The drawing under review shows one solid part. Ordinate dimensions are in mm from its lowest x, y, z. A direction names the side the tool comes from. Coordinates: 2 decimals unless noted, no trailing zeros. Order: outer loops, then holes, each group sorted by start corner. A loop starts at its lowest first (then second) coordinate and runs counter-clockwise, first axis right, second up. Notation, with made-up numbers: (23.25, 23.5) - (72.25, 23.5) arc R15 ccw to (72.25, 46.5) - close; hole circle Ø7 at (-14, 61.5). An arc over 180 degrees is marked (long way). Write each question's results on one line, items separated by ' | '. Start each with the question number.
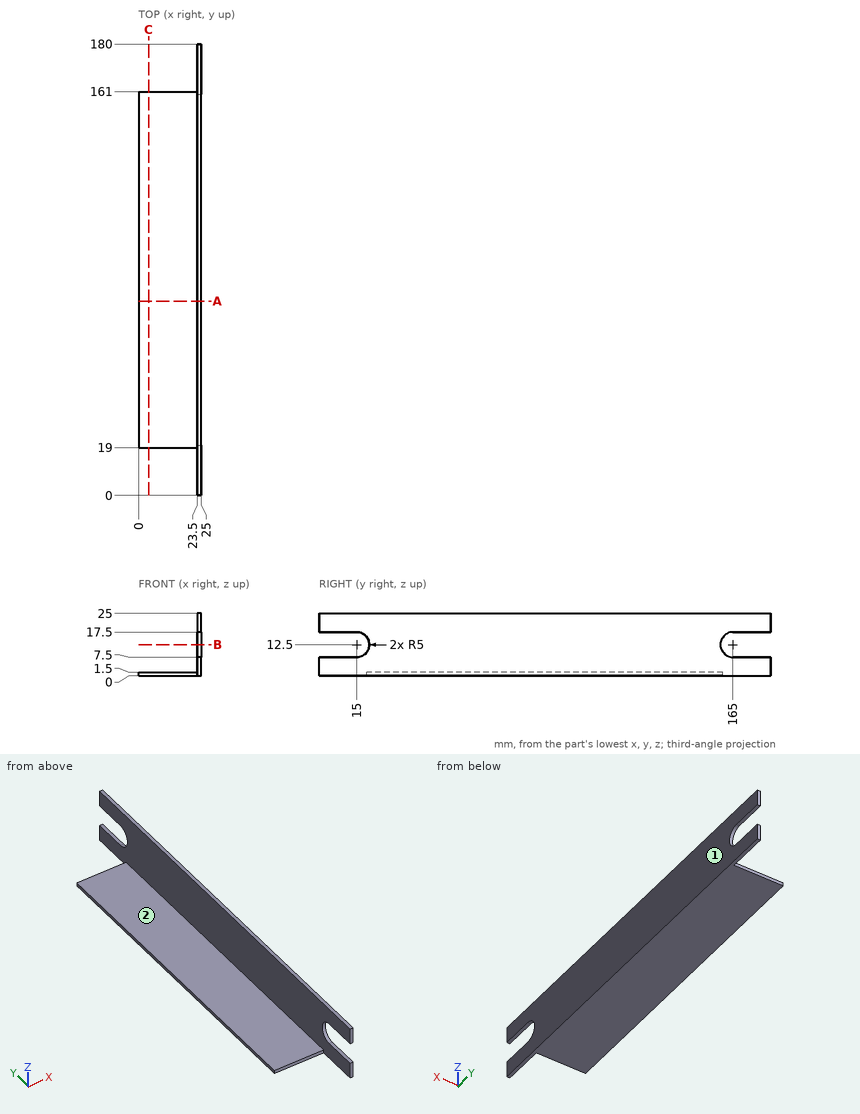
(1) Take a section at B-B (z = 12.5). State the section outline as (x, y) points.
(2) Tool access review of the marked faces 1 and 2: name each direction out of +Z, -Z, +X, -X, +Y, -Y from which nothing blocks a thin tool from reaching the whole face with its end or side.
(3) To check wall thickness, follow line 1 along Z through (x, y) = (6, 127); line 2 along X through (y, z) = (132.5, 13.5). State the ranges of each line that lie inside material, in increasing order. Write a range as [from, to].
(4) Clearance check with flat-ended pins moving along their axes: pin 1 (0.8 mm diameter, centred on x = 24, y = 172.5, fed in from -Z); pin 2 (6 mm diameter, centred on y = 94.5, z = 8.5, fed in from -X); pin 3 (0.8 mm diameter, centred on x = 13.5, z = 1, fed in from +Y); pin 4 (1.6 mm diameter, centred on x = 16, z = 1, fed in from -Y). State where each tip first meets the part, or that it passes through.
(5) Take a section at C-C (x = 4). State the section outline as (y, z) points.
(6) Take a section at A-A (y = 77.5). State the section outline as (x, z) points, plus the area to 4 significant figures.
Worked out:
1) outline: (23.5, 20) - (25, 20) - (25, 160) - (23.5, 160) - close
2) face 1: +Z, -Z, +X, +Y, -Y | face 2: +Z, -X, +Y, -Y
3) line 1: [0, 1.5] | line 2: [23.5, 25]
4) pin 1: z = 0 | pin 2: x = 23.5 | pin 3: y = 161 | pin 4: y = 19
5) outline: (19, 0) - (161, 0) - (161, 1.5) - (19, 1.5) - close
6) outline: (0, 0) - (25, 0) - (25, 25) - (23.5, 25) - (23.5, 1.5) - (0, 1.5) - close | area: 72.75 mm^2
